Verification items for the finished model (mm, model axes). A direction names the side the tool comes from. Give positions to 0.01 mm unless a question says otherwise; leave off trailing zeros. Order: outer loops, then holes, each group sorted by start corner. A loop starts at its lowest first (then second) coordinate and runs counter-clockwise, first axis right, second up. Notation, with made-up numbers: M -20,30.25 L -6,30.25 A19 cw -6,64.25 Z; hole C -18,3.5 d10. An arc over 180 degrees is marked long. Answer as a JSON object with one key per item and string values.
```python
from build123d import *

# Parameters (mm, degrees)
SKETCH1_W           = 120
SKETCH1_H           = 41
BOSS_EXTRUDE1_DEPTH = 250
CUT_EXTRUDE1_DEPTH  = 250
SKETCH3_R           = 6
CUT_EXTRUDE2_DEPTH  = 250


with BuildPart() as part:
    # Sketch1 → Boss-Extrude1 (new body)
    with BuildSketch(Plane(origin=(0, 0, 0), x_dir=(1, 0, 0), z_dir=(0, 1, 0))):
        Rectangle(SKETCH1_W, SKETCH1_H)
    extrude(amount=BOSS_EXTRUDE1_DEPTH)

    # Sketch2 → Cut-Extrude1 (cut)
    with BuildSketch(Plane(origin=(0, 250, 0), x_dir=(1, 0, 0), z_dir=(0, 1, 0))):
        Polygon((-36, 20.5), (-44.948929172, 5), (39.708929172, 5), (30.76, 20.5), align=None)
    extrude(amount=-CUT_EXTRUDE1_DEPTH, mode=Mode.SUBTRACT)

    # Sketch3 → Cut-Extrude2 (cut)
    with BuildSketch(Plane.XY.offset(20.5)):
        with Locations((0, 150)):
            Circle(SKETCH3_R)
    extrude(amount=-CUT_EXTRUDE2_DEPTH, mode=Mode.SUBTRACT)


solid = part.part
```
Q1. Section check B-B on y = 150. Record the cut outline in (x, z).
Resolved:
{"outline": "M -60,-20.5 L -36,-20.5 L -44.95,-5 L -6,-5 L -6,20.5 L -60,20.5 Z; M 6,-5 L 39.71,-5 L 30.76,-20.5 L 60,-20.5 L 60,20.5 L 6,20.5 Z"}
Q2. Tool access check on faces 5 (the face through (-40.41, 126.75, -12.86)), 6 (the face through (-48, 123, -20.5)). Record the directions out of +Z, -Z, +X, -X, +Y, -Y that give a thin tool (end or side, any length) a straight path to the whole face; none if there is none.
Resolved:
{"face 5": "+Y, -Y", "face 6": "-Z, +X, -X, +Y, -Y"}
Q3. Release check for a two-part mould opening along Y. For faces 1 (the face through (-1, 250, 4)), 2 (the face through (-1.301, 144.143, 7.928)), 3 (the face through (-1, 0, 4)), 4 (the face through (-1, 123, 20.5)) record: +Y half, -Y half, draft (parallel to the pull), parting line (faces both ways), or undercut.
Resolved:
{"face 1": "+Y half", "face 2": "undercut", "face 3": "-Y half", "face 4": "draft"}
Q4. Gauge pin test, flat ends, axial feed: pin 1 Ø10 at (x, y) = (24, 91) entering from -Z; pin 2 Ø9.5 at (x, y) = (0, 150) entering from -Z. Record the tip position at first contact, or that the pin passes through.
Resolved:
{"pin 1": "stops at z = -5", "pin 2": "passes through"}
Q5. Section check A-A on x = 0. Record the cut outline in (y, z).
Resolved:
{"outline": "M 0,-5 L 144,-5 L 144,20.5 L 0,20.5 Z; M 156,-5 L 250,-5 L 250,20.5 L 156,20.5 Z"}
Q6. Section check D-D on x = -18.5. Record the cut outline in (y, z), then the cut area to 4 significant figures.
Resolved:
{"outline": "M 0,-5 L 250,-5 L 250,20.5 L 0,20.5 Z", "area": "6,375 mm²"}
Q7. Section check C-C on y = 87. Record the cut outline in (x, z), then the cut area to 3 significant figures.
Resolved:
{"outline": "M -60,-20.5 L -36,-20.5 L -44.95,-5 L 39.71,-5 L 30.76,-20.5 L 60,-20.5 L 60,20.5 L -60,20.5 Z", "area": "3,750 mm²"}
Q8. Material ranges on L1, parallel to Y at x = 0, z = 8.5; L2, parallel to Z at x = -10, y = 236; L3, parallel to X at y = 202.5, z = -15, recorded low to high.
Resolved:
{"L1": "y = 0 to 144, 156 to 250", "L2": "z = -5 to 20.5", "L3": "x = -60 to -39.18, 33.94 to 60"}
